The listing builds one solid part. Answer for the finished solid, in the listing's coordinates (mm). A direction names the side the tool comes from. Round coordinates to 2 decimals unless told otherwise and drop trailing zeros. Write each loop counter-clockwise with the first axis right and the second up, starting at its lowest first coordinate (ties: lowest second). Pieces come first, ordered by that corner, then holes.
from build123d import *

# Parameters (mm, degrees)
BOSS_EXTRUDE1_DEPTH            = 50
F_3_2_3_2_DIAMETER_HOLE1_D     = 3.2
F_3_2_3_2_DIAMETER_HOLE1_DEPTH = 7
SKETCH5_R                      = 2.25
CUT_EXTRUDE1_DEPTH             = 71.434810286
SKETCH6_W                      = 15
SKETCH6_H                      = 4.75
BOSS_EXTRUDE2_DEPTH            = 26
SKETCH8_W                      = 12.2
SKETCH8_H                      = 15
BOSS_EXTRUDE3_DEPTH            = 25
SKETCH9_R                      = 2.75
CUT_EXTRUDE2_DEPTH             = 96.990220856
BOSS_EXTRUDE4_DEPTH            = 26
CUT_EXTRUDE3_REACH             = 99.075
SKETCH11_R                     = 2.75


with BuildPart() as part:
    # Sketch1 → Boss-Extrude1 (new body)
    with BuildSketch(Plane.XY):
        Polygon((-10.5, 0), (15.5, 0), (15.5, 42.25), (-10.5, 42.25), (-10.5, 37.5), (10.5, 37.5), (10.5, 7), (-10.5, 7), align=None)
    extrude(amount=BOSS_EXTRUDE1_DEPTH)

    # Ø3.2 (3.2) Diameter Hole1
    with Locations(Plane(origin=(0, 0, 0), x_dir=(-1, 0, 0), z_dir=(0, -1, 0))):
        with Locations((-7.5, -17), (7.5, -17), (7.5, -33), (-7.5, -33)):
            Hole(F_3_2_3_2_DIAMETER_HOLE1_D / 2, depth=F_3_2_3_2_DIAMETER_HOLE1_DEPTH)

    # Sketch5 → Cut-Extrude1 (cut, through all)
    with BuildSketch(Plane(origin=(15.5, 0, 0), x_dir=(0, 0, -1), z_dir=(1, 0, 0))):
        with Locations(Location((-37, 32.25, 0), (0, 0, 90))):
            Circle(SKETCH5_R)
        with Locations(Location((-13, 32.25, 0), (0, 0, 90))):
            Circle(SKETCH5_R)
        with Locations(Location((-37, 15.25, 0), (0, 0, 90))):
            Circle(SKETCH5_R)
        with Locations(Location((-13, 15.25, 0), (0, 0, 90))):
            Circle(SKETCH5_R)
    extrude(amount=-CUT_EXTRUDE1_DEPTH, mode=Mode.SUBTRACT)

    # Sketch6 → Boss-Extrude2 (add)
    with BuildSketch(Plane(origin=(15.5, 0, 0), x_dir=(0, 0, -1), z_dir=(1, 0, 0))):
        with Locations((-57.5, 39.875)):
            Rectangle(SKETCH6_W, SKETCH6_H)
        with Locations((7.5, 39.875)):
            Rectangle(SKETCH6_W, SKETCH6_H)
    extrude(amount=-BOSS_EXTRUDE2_DEPTH)

    # Sketch8 → Boss-Extrude3 (add)
    with BuildSketch(Plane(origin=(0, 42.25, 0), x_dir=(1, 0, 0), z_dir=(0, 1, 0))):
        with Locations((0, 7.5)):
            Rectangle(SKETCH8_W, SKETCH8_H)
        with Locations((0, -57.5)):
            Rectangle(SKETCH8_W, SKETCH8_H)
    extrude(amount=BOSS_EXTRUDE3_DEPTH)

    # Sketch9 → Cut-Extrude2 (cut, through all)
    with BuildSketch(Plane.ZY.offset(6.1)):
        with Locations((-7.5, 54.45)):
            Circle(SKETCH9_R)
        with Locations((57.5, 54.45)):
            Circle(SKETCH9_R)
    extrude(amount=-CUT_EXTRUDE2_DEPTH, mode=Mode.SUBTRACT)

    # Sketch10 → Boss-Extrude4 (add)
    with BuildSketch(Plane.ZY.offset(10.5)):
        with BuildLine():
            Line((11.196152423, -3), (12.92820323, 0))
            Line((12.92820323, 0), (0, 0))
            ThreePointArc((0, 0), (4.447085729, -5.795554958), (11.196152423, -3))
        make_face()
        with BuildLine():
            Line((22, 50.196152423), (8.236860279, 42.25))
            Line((8.236860279, 42.25), (41.763139721, 42.25))
            Line((41.763139721, 42.25), (28, 50.196152423))
            ThreePointArc((28, 50.196152423), (25, 51), (22, 50.196152423))
        make_face()
        with BuildLine():
            Line((38.803847577, -3), (37.07179677, 0))
            Line((37.07179677, 0), (50, 0))
            ThreePointArc((50, 0), (45.552914271, -5.795554958), (38.803847577, -3))
        make_face()
    extrude(amount=-BOSS_EXTRUDE4_DEPTH)

    # Sketch11 → Cut-Extrude3 (cut, up to next)
    with BuildSketch(Plane.ZY.offset(10.5), mode=Mode.PRIVATE) as cut_extrude3_sk1:
        with Locations(Location((25, 45, 0), (0, 0, 270))):
            Circle(SKETCH11_R)
    cut_extrude3_tool1 = extrude(cut_extrude3_sk1.sketch, amount=-CUT_EXTRUDE3_REACH, mode=Mode.PRIVATE) & part.part
    # Sketch11 → Cut-Extrude3 (cut, up to next)
    with BuildSketch(Plane.ZY.offset(10.5), mode=Mode.PRIVATE) as cut_extrude3_sk2:
        with Locations(Location((44, 0, 0), (0, 0, 270))):
            Circle(SKETCH11_R)
    cut_extrude3_tool2 = extrude(cut_extrude3_sk2.sketch, amount=-CUT_EXTRUDE3_REACH, mode=Mode.PRIVATE) & part.part
    # Sketch11 → Cut-Extrude3 (cut, up to next)
    with BuildSketch(Plane.ZY.offset(10.5), mode=Mode.PRIVATE) as cut_extrude3_sk3:
        with Locations(Location((6, 0, 0), (0, 0, 270))):
            Circle(SKETCH11_R)
    cut_extrude3_tool3 = extrude(cut_extrude3_sk3.sketch, amount=-CUT_EXTRUDE3_REACH, mode=Mode.PRIVATE) & part.part
    add(cut_extrude3_tool1.solids().sort_by_distance((-10.5, 45, 25))[0], mode=Mode.SUBTRACT)
    add(cut_extrude3_tool2.solids().sort_by_distance((-10.5, 0, 44))[0], mode=Mode.SUBTRACT)
    add(cut_extrude3_tool3.solids().sort_by_distance((-10.5, 0, 6))[0], mode=Mode.SUBTRACT)


solid = part.part
1. Given pin 1 (5 mm diameter, centred on x = 7.5, z = 33, fed in from -Y); pin 2 (1.5 mm diameter, centred on x = 12, z = 25, fed in from +Y); pin 3 (12 mm diameter, centred on y = 49.5, z = -8, fed in from +X); pin 4 (5 mm diameter, centred on y = 0, z = 6, fed in from +X), each flat-ended and moving along its own axis, determine where each tip first touches the part or whether it passes through.
Geometry says:
pin 1: stops at y = 0
pin 2: stops at y = 51
pin 3: stops at x = 6.1
pin 4: passes through
2. For a pull along Z with two mould halves and no side action, classify faces 5 (the face through (13.035, 16.46, 38.897)), 6 (the face through (0, 7, 25)), 7 (the face through (0, 52, -15)) as released by +Z, released by -Z, zero draft, split by the parting line, or undercut.
Geometry says:
face 5: undercut
face 6: zero draft
face 7: released by -Z
3. Section D-D on x = -5 is taken. Determine the outline of the cut face in (y, z).
Geometry says:
outline: (-3, 11.2) arc R6 ccw to (0, 0) - (7, 0) - (7, 50) - (0, 50) arc R6 ccw to (-3, 38.8) - (0, 37.07) - (0, 12.93) - close; (37.5, -15) - (67.25, -15) - (67.25, 0) - (42.25, 0) - (42.25, 8.24) - (50.2, 22) arc R6 ccw to (50.2, 28) - (42.25, 41.76) - (42.25, 50) - (67.25, 50) - (67.25, 65) - (37.5, 65) - close; hole circle Ø5.5 at (0, 6); hole circle Ø5.5 at (0, 44); hole circle Ø5.5 at (45, 25); hole circle Ø5.5 at (54.45, -7.5); hole circle Ø5.5 at (54.45, 57.5)
4. Section B-B on y = 45 is taken. Determine the outline of the cut face in (x, z), plus the area to 3 significant figures.
Geometry says:
outline: (-10.5, 13) - (15.5, 13) - (15.5, 22.25) - (-10.5, 22.25) - close; (-10.5, 27.75) - (15.5, 27.75) - (15.5, 37) - (-10.5, 37) - close; (-6.1, -15) - (6.1, -15) - (6.1, 0) - (-6.1, 0) - close; (-6.1, 50) - (6.1, 50) - (6.1, 65) - (-6.1, 65) - close
area: 847 mm2
5. Section A-A on x = 7.5 is taken. Determine the outline of the cut face in (y, z), plus the area to 3 significant figures.
Geometry says:
outline: (-3, 11.2) arc R6 ccw to (0, 0) - (7, 0) - (7, 15.4) - (0, 15.4) - (0, 12.93) - close; (-3, 38.8) - (0, 37.07) - (0, 34.6) - (7, 34.6) - (7, 50) - (0, 50) arc R6 ccw to start; (0, 18.6) - (7, 18.6) - (7, 31.4) - (0, 31.4) - close; (37.5, -15) - (42.25, -15) - (42.25, 8.24) - (50.2, 22) arc R6 ccw to (50.2, 28) - (42.25, 41.76) - (42.25, 65) - (37.5, 65) - close; hole circle Ø5.5 at (0, 6); hole circle Ø5.5 at (0, 44); hole circle Ø5.5 at (45, 25)
area: 889 mm2
6. Straight lines are drawn through the part: line 1 along Z through (x, y) = (-7.5, 5); line 2 along Z through (x, y) = (13.4, 15.25); line 3 along X through (y, z) = (5, 17). For each, find the intervals that lie inside material, in ascending order.
Geometry says:
line 1: z = 0 to 15.4, 18.6 to 31.4, 34.6 to 50
line 2: z = 0 to 10.75, 15.25 to 34.75, 39.25 to 50
line 3: x = -10.5 to -9.1, -5.9 to 5.9, 9.1 to 15.5
7. Section C-C on z = 6 is taken. Determine the outline of the cut face in (x, y).
Geometry says:
outline: (-10.5, -6) - (15.5, -6) - (15.5, -2.75) - (-10.5, -2.75) - close; (-10.5, 2.75) - (15.5, 2.75) - (15.5, 42.25) - (-10.5, 42.25) - (-10.5, 37.5) - (10.5, 37.5) - (10.5, 7) - (-10.5, 7) - close
8. A tool of negligible diameter and unlimited length cuts with its end or side. For faces 1 (the face through (2.318, 46.167, 34.978)), 2 (the face through (6.1, 57.4, 57.6)), 3 (the face through (2.32, -1.52, 37.95)), 4 (the face through (-7.708, 3.549, 15.414)), from which of +Z, -Z, +X, -X, +Y, -Y can it reach the whole face along a straight path? Write none if from no direction.
Geometry says:
face 1: +X, -X, +Y
face 2: +Z, +X, +Y
face 3: +X, -X, -Y
face 4: -Y
